CAD build for the part. Positions are in the model's coordinates, mm. A direction names the side the tool comes from. Round coordinates to 2 decimals unless told otherwise and drop trailing zeros. Order: outer loops, then holes, each group sorted by start corner. A loop starts at its lowest first (then second) coordinate and runs counter-clockwise, first axis right, second up. Notation, with made-up numbers: M 22,85.5 L 48,85.5 A26 cw 48,108.5 Z; hole C -30,14.5 d3. An arc over 180 degrees is marked long. Answer as a JSON object with one key per item and string values.
```python
from build123d import *

# Parameters (mm, degrees)
SKETCH1_W           = 5.5
SKETCH1_H           = 39.3
BOSS_EXTRUDE1_DEPTH = 1
SKETCH3_W           = 20
SKETCH3_H           = 26
BOSS_EXTRUDE5_DEPTH = 1
CUT_EXTRUDE3_DEPTH  = 1
SKETCH5_W           = 5
SKETCH5_H           = 23
CUT_EXTRUDE4_DEPTH  = 1


with BuildPart() as part:
    # Sketch1 → Boss-Extrude1 (new body)
    with BuildSketch(Plane.XY):
        Rectangle(SKETCH1_W, SKETCH1_H)
    extrude(amount=BOSS_EXTRUDE1_DEPTH)

    # Sketch3 → Boss-Extrude5 (add)
    with BuildSketch(Plane.XY.offset(1)):
        with Locations((-7.25, 11.4)):
            Rectangle(SKETCH3_W, SKETCH3_H)
    extrude(amount=-BOSS_EXTRUDE5_DEPTH)

    # Sketch4 → Cut-Extrude3 (cut)
    with BuildSketch(Plane.XY.offset(1)):
        with BuildLine():
            Line((-14.56, 22.9), (-14.54, 22.9))
            ThreePointArc((-14.54, 22.9), (-13.69854293, 22.55145707), (-13.35, 21.71))
            Line((-13.35, 21.71), (-13.35, 1.09))
            ThreePointArc((-13.35, 1.09), (-13.69854293, 0.24854293), (-14.54, -0.1))
            Line((-14.54, -0.1), (-14.56, -0.1))
            ThreePointArc((-14.56, -0.1), (-15.40145707, 0.24854293), (-15.75, 1.09))
            Line((-15.75, 1.09), (-15.75, 21.71))
            ThreePointArc((-15.75, 21.71), (-15.40145707, 22.55145707), (-14.56, 22.9))
        make_face()
    extrude(amount=-CUT_EXTRUDE3_DEPTH, mode=Mode.SUBTRACT)

    # Sketch5 → Cut-Extrude4 (cut)
    with BuildSketch(Plane.XY.offset(1)):
        with Locations((-1.25, 11.4)):
            Rectangle(SKETCH5_W, SKETCH5_H)
    extrude(amount=-CUT_EXTRUDE4_DEPTH, mode=Mode.SUBTRACT)


solid = part.part
```
Item 1: Saw through at D-D on x = -15. List the corners of the cut face in (y, z), and give its area (3 significant figures).
Worked answers:
{"outline": "M -1.6,0 L -0.02,0 L -0.02,1 L -1.6,1 Z; M 22.82,0 L 24.4,0 L 24.4,1 L 22.82,1 Z", "area": "3.17 mm2"}
Item 2: Drop a flat-ended pin along its axis: pin 1 Ø5 at (x, y) = (-7, 7) entering from -Z. Give the stop position or say it passes through.
Worked answers:
{"pin 1": "stops at z = 0"}
Item 3: 3-axis set-ups, long thin cutter, end or side, ignore diameter. For faces 4 (the flat face through (-15.75, 11.3, 0.5)), 5 (the flat face through (-10.1, -1.6, 0.5)), 6 (the flat face through (0, -19.65, 0.5)): which of +Z, -Z, +X, -X, +Y, -Y reach the whole face in a straight line?
Worked answers:
{"face 4": "+Z, -Z", "face 5": "+Z, -Z, -X, -Y", "face 6": "+Z, -Z, +X, -X, -Y"}
Item 4: Wall check: line 1 along X through (y, z) = (13.5, 0.3); line 2 along Y through (x, z) = (-1.5, 0.2); line 3 along X through (y, z) = (-10, 0.5). Give the ranges that are in metal, low to high. Write a range as [from, to].
Worked answers:
{"line 1": "x = [-17.25, -15.75], [-13.35, -3.75], [1.25, 2.75]", "line 2": "y = [-19.65, -0.1], [22.9, 24.4]", "line 3": "x = [-2.75, 2.75]"}
Item 5: Two-plate mould, pull along X, no slides. Class faces 1 (the flat face through (1.25, 11.2, 0.5)), 2 (the flat face through (-7, 8, 1)), 3 (the flat face through (-2.75, -10.8, 0.5)): released by +X, released by -X, zero draft, split by the parting line, or undercut.
Worked answers:
{"face 1": "undercut", "face 2": "zero draft", "face 3": "released by -X"}
Item 6: Saw through at C-C on x = -1. List the corners of the cut face in (y, z), and give its area (4 significant figures).
Worked answers:
{"outline": "M -19.65,0 L -0.1,0 L -0.1,1 L -19.65,1 Z; M 22.9,0 L 24.4,0 L 24.4,1 L 22.9,1 Z", "area": "21.05 mm2"}
Item 7: Saw through at B-B on y = 10.5. List the corners of the cut face in (x, z).
Worked answers:
{"outline": "M -17.25,0 L -15.75,0 L -15.75,1 L -17.25,1 Z; M -13.35,0 L -3.75,0 L -3.75,1 L -13.35,1 Z; M 1.25,0 L 2.75,0 L 2.75,1 L 1.25,1 Z"}
Item 8: Saw through at A-A on z = 0.85. State how many separate pieces and enclosed holes the cut face has, and give its area (3 significant figures).
Worked answers:
{"separate pieces": "1", "enclosed holes": "2", "area": "450 mm2"}
